Here's how the part is built. I have some questions about the finished solid (model axes, mm). A direction names the side the tool comes from. Coordinates: 2 decimals unless noted, no trailing zeros. Write each loop counter-clockwise with the first axis right and the second up, starting at its lowest first coordinate (ties: lowest second). Pieces come first, ordered by that corner, then holes.
Item 1: I want a section at B-B (y = 19). Please give me the cut outline in (x, z).
Item 2: I want a section at D-D (z = 11). Please give me the cut outline in (x, y), and give its area (3 significant figures).
Item 3: For faces 1 (the face through (1.07, 11.38, -8.13)), 2 (the face through (-1.07, 45.96, 8.13)), 3 (the face through (-9.999, 28.751, -7.667)), which set-ups out of +Z, -Z, +X, -X, +Y, -Y let a thin tool reach every point of the face, with its end or its side?
Item 4: I want a section at C-C (z = -2.5). Please give me the cut outline in (x, y).
Item 5: Please list where these lines run through material, in increasing order: line 1 (Z direction, x = 0, y = 47); line 2 (Y direction, x = -7, z = -4.5).
Item 6: I'm going to push flat-ended pins straight in: P1, Ø12, axis at y = 48.5, z = -4, coming from the +X side; P2, Ø1, axis at x = -3, z = -6, coming from the +Y side; P3, Ø8, axis at x = 9, y = 46.5, coming from the -Z side; P4, Ø1, axis at x = 8.5, z = 6.5, coming from the +Y side. Where does each tip first touch, or does it pass through?
Autodesk Inventor part; units mm, degrees
ref_plane "YZ Plane" through (0, 0, 0) normal (1, 0, 0) x (0, 1, 0)
ref_plane "XZ Plane" through (0, 0, 0) normal (0, 1, 0) x (-1, 0, 0)
ref_plane "XY Plane" through (0, 0, 0) normal (0, 0, 1) x (1, 0, 0)
sketch "Sketch1" plane through (0, 0, 0) normal (0, 1, 0) x (-1, 0, 0)
  circle A0 centre (0, 0) radius 7.7
  circle A1 centre (0, 0) radius 8.2
  dimension "d0" = 15.4
  dimension "d1" = 16.4
extrude "Extrusion1" add sketch "Sketch1" along normal blind 23.0816
sketch "Sketch2" plane through (0, 23.0816, 0) normal (0, 1, 0) x (1, 0, 0)
  circle A0 centre (0, 0) radius 12.6
  circle A1 centre (0, 0) radius 7.7
  dimension "d4" = 25.2
extrude "Extrusion2" add sketch "Sketch2" along normal blind 11.5
sketch "Sketch3" plane through (0, 34.5816, 0) normal (0, 1, 0) x (1, 0, 0)
  circle A0 centre (0, 0) radius 8.2
  circle A1 centre (0, 0) radius 7.7
extrude "Extrusion3" add sketch "Sketch3" along normal blind 23.0816
equation "\"delta\" = 7.0816"
properties part number "ICF34_Ceramic" material "Stainless Steel, 440C"
Answer:
1. outline: circle Ø16.4 at (0, 0); hole circle Ø15.4 at (0, 0)
2. outline: (-6.14, 23.08) - (6.14, 23.08) - (6.14, 34.58) - (-6.14, 34.58) - close
2. area: 141 mm2
3. face 1: -Y
3. face 2: +Y
3. face 3: +Y, -Y
4. outline: (-12.35, 23.08) - (-7.81, 23.08) - (-7.81, 0) - (-7.28, 0) - (-7.28, 57.66) - (-7.81, 57.66) - (-7.81, 34.58) - (-12.35, 34.58) - close; (7.28, 0) - (7.81, 0) - (7.81, 23.08) - (12.35, 23.08) - (12.35, 34.58) - (7.81, 34.58) - (7.81, 57.66) - (7.28, 57.66) - close
5. line 1: z = -8.2 to -7.7, 7.7 to 8.2
5. line 2: y = 23.08 to 34.58
6. P1: stops at x = 8.2
6. P2: passes through
6. P3: stops at z = -6.5
6. P4: stops at y = 34.58
